Can you work these out from the drawing? Everything is in mm from the part's minimum corner. Coordinates: 2 decimals unless noted, no trailing zeros. Order: outer loops, then holes, each group sorted by start corner. A loop starts at its lowest first (then second) coordinate and runs counter-clockwise, first axis right, second up. Notation, with made-up numbers: (-20, 1.5) -> (-12, 1.5) arc R13 ccw to (-12, 22.5) -> close; hole circle Ø8 at (-13, 76). An arc over 180 degrees is marked (long way). Use a Markdown table: item, result. Add a question column.
1) If we section it at D-D (y = 5): Write out the boundary of the cut face in (x, z), plus the area to 3 significant figures.
2) If I drill on L1, parallel to Y at x = 25, z = 0.95 (3 decimals); L2, parallel to Y at x = 31.5, z = 0.35; L3, parallel to X at y = 4, z = 2.6 (1 decimal), over which ranges is the centre line in solid material (lowest first)? Write a range as [from, to].
3) If we section it at C-C (z = 1.65): Give the number of separate pieces and of enclosed holes in the cut face, plus the area to 3 significant figures.
4) If we section it at A-A (x = 25): Write out the boundary of the cut face in (y, z) (3 decimals).
5) Will these pins go through, and if not, where does the flat tip stop? pin 1 Ø3 at (x, y) = (43.5, 19.5) entering from -Z; pin 2 Ø1.2 at (x, y) = (47.715, 25) entering from -Z.
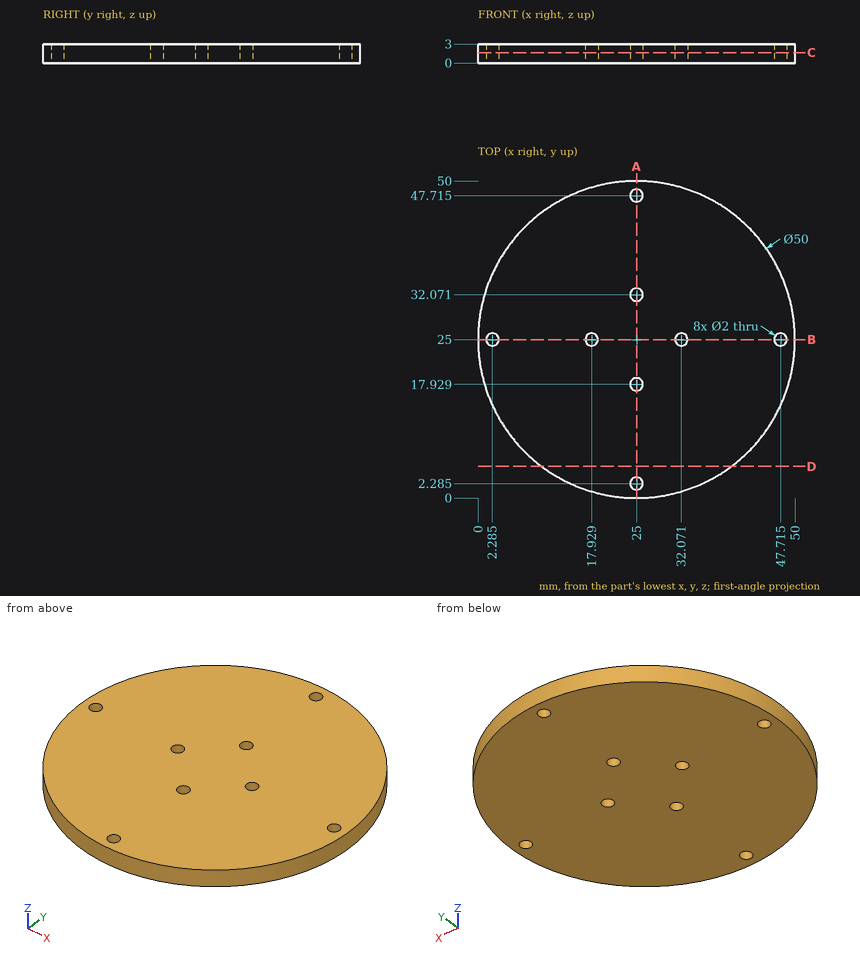
Answer sheet:
| question | item | result |
|---|---|---|
| 1 | outline | (10, 0) -> (40, 0) -> (40, 3) -> (10, 3) -> close |
| 1 | area | 90.0 mm2 |
| 2 | L1 | [0, 1.285], [3.285, 16.929], [18.929, 31.071], [33.071, 46.715], [48.715, 50] |
| 2 | L2 | [0.86, 24.18], [25.82, 49.14] |
| 2 | L3 | [11.4, 38.6] |
| 3 | separate pieces | 1 |
| 3 | enclosed holes | 8 |
| 3 | area | 1,940 mm2 |
| 4 | outline | (0, 0) -> (1.285, 0) -> (1.285, 3) -> (0, 3) -> close; (3.285, 0) -> (16.929, 0) -> (16.929, 3) -> (3.285, 3) -> close; (18.929, 0) -> (31.071, 0) -> (31.071, 3) -> (18.929, 3) -> close; (33.071, 0) -> (46.715, 0) -> (46.715, 3) -> (33.071, 3) -> close; (48.715, 0) -> (50, 0) -> (50, 3) -> (48.715, 3) -> close |
| 5 | pin 1 | z = 0 |
| 5 | pin 2 | through |
